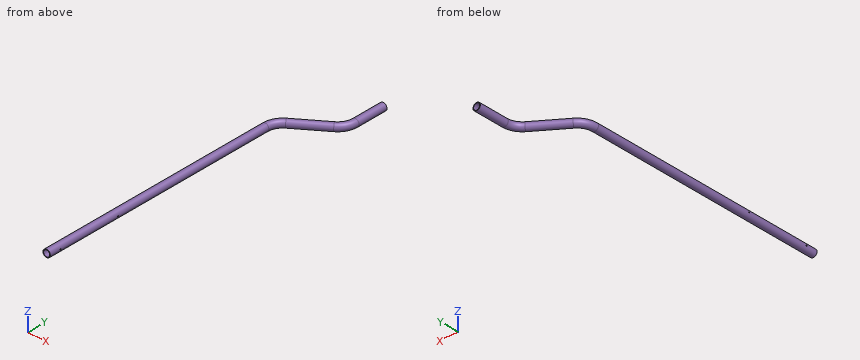
```python
from build123d import *

# Parameters (mm, degrees)
SKETCH3_R               = 21.082
SKETCH3_R_2             = 17.526
SKETCH5_R               = 3.3734375
CUT_EXTRUDE1_DEPTH      = 276.0820001
CUT_EXTRUDE1_DEPTH_BACK = 22.0820001


with BuildPart() as part:
    # Sweep1: sweep along a path in Sketch2
    with BuildLine(Plane.XY) as sweep1_path:
        Line((0, 0), (0, 1350.407672959))
        ThreePointArc((0, 1350.407672959), (11.479699349, 1397.321332063), (43.324634067, 1433.633520658))
        Line((43.324634067, 1433.633520658), (210.675365933, 1550.813764636))
        ThreePointArc((210.675365933, 1550.813764636), (242.520300651, 1587.125953231), (254, 1634.039612336))
        Line((254, 1634.039612336), (254, 1806.575))
    # Sketch3 → Sweep1 (sweep)
    with BuildSketch(Plane(origin=(0, 1806.575, 0), x_dir=(1, 0, 0), z_dir=(0, 1, 0))):
        with Locations((254, 0)):
            Circle(SKETCH3_R)
        with Locations((254, 0)):
            Circle(SKETCH3_R_2, mode=Mode.SUBTRACT)
    sweep(path=sweep1_path.line)

    # Sketch5 → Cut-Extrude1 (cut, two sides)
    with BuildSketch(Plane(origin=(0, 0, 0), x_dir=(0, 0, -1), z_dir=(1, 0, 0))) as cut_extrude1_sk:
        with Locations((0, 63.5)):
            Circle(SKETCH5_R)
        with Locations((0, 419.1)):
            Circle(SKETCH5_R)
    extrude(amount=CUT_EXTRUDE1_DEPTH, mode=Mode.SUBTRACT)
    extrude(cut_extrude1_sk.sketch, amount=-CUT_EXTRUDE1_DEPTH_BACK, mode=Mode.SUBTRACT)


solid = part.part
```
Here's how the part is built. I have some questions about the finished solid (model axes, mm). Round coordinates to 2 decimals unless told otherwise and drop trailing zeros. Write each loop counter-clockwise with the first axis right and the second up, starting at its lowest first coordinate (ties: lowest second). Pieces come first, ordered by that corner, then holes. Notation, with made-up numbers: M 56,76.5 L 69,76.5 A25 ccw 69,114.5 Z; hole C 59.5,58 d5. An arc over 180 degrees is marked long. Answer as CSV lines item,"result". Start each with the question number.
1. I need wall thicknesses on probe 1 along X at (y, z) = (1723.5, 0); probe 2 along X at (y, z) = (920.5, 2); probe 3 along Z at (x, y) = (-18, 63) (3 decimals). Which ranges of each line are inside material? Lowest first, please.
2. Suppose I cut it at A-A on y = 1192. Write out the boundary of the cut face in (x, z).
3. I'm going to push flat-ended pins straight in: pin 1 Ø2 at (y, z) = (531.5, 14) entering from +X; pin 2 Ø4 at (x, z) = (155, -8.5) entering from +Y; pin 3 Ø8 at (y, z) = (419.1, 0) entering from +X; pin 4 Ø10 at (y, z) = (1079.5, 3) entering from -X. Where does each tip first touch, or does it pass through?
Check result:
1,probe 1,"x = 232.92 to 236.47, 271.53 to 275.08"
1,probe 2,"x = -20.99 to -17.41, 17.41 to 20.99"
1,probe 3,"z = -10.975 to -3.336, 3.336 to 10.975"
2,outline,"C 0,0 d42.16; hole C 0,0 d35.05"
3,pin 1,"stops at x = 16.6"
3,pin 2,"stops at y = 1537.1"
3,pin 3,"stops at x = 21.08"
3,pin 4,"stops at x = -21.08"
